from build123d import *

# Parameters (mm, degrees)
CYLINDER178_R          = 3
CYLINDER178_DEPTH      = 62
CYLINDER179_R          = 3
CYLINDER179_DEPTH      = 62
CYLINDER174_R          = 1.2
CYLINDER174_DEPTH      = 4
CYLINDER176_R          = 1.2
CYLINDER176_DEPTH      = 8
CYLINDER177_R          = 1.2
CYLINDER177_DEPTH      = 8
CYLINDER175_R          = 1.2
CYLINDER175_DEPTH      = 4
CYLINDER002_R          = 1.6
CYLINDER002_DEPTH      = 41
CYLINDER003_R          = 2.6
CYLINDER003_DEPTH      = 20
CYLINDER001_R          = 1.4
CYLINDER001_DEPTH      = 51
CYLINDER008_R          = 1.25
CYLINDER008_DEPTH      = 15
CYLINDER007_R          = 1.25
CYLINDER007_DEPTH      = 15
CYLINDER009_R          = 1.25
CYLINDER009_DEPTH      = 15
CYLINDER005_R          = 1.25
CYLINDER005_DEPTH      = 15
CYLINDER006_R          = 1.25
CYLINDER006_DEPTH      = 15
CYLINDER004_R          = 1.25
CYLINDER004_DEPTH      = 15
CYLINDER_R             = 5
CYLINDER_DEPTH         = 19
BOX084_W               = 30
BOX084_H               = 62
BOX084_DEPTH           = 10
BOX084_PLACEMENT_ANGLE = 17
BOX083_W               = 25
BOX083_H               = 42
BOX083_DEPTH           = 1.5
BOX079_W               = 25
BOX079_H               = 62
BOX079_DEPTH           = 11
FILLET045_R            = 3
BOX008_W               = 60
BOX008_H               = 60
BOX008_DEPTH           = 10
FILLET044_R            = 3
FILLET046_R            = 3


with BuildPart() as cylinder178:
    # Cylinder178 → Cylinder178 (new body)
    with BuildSketch(Plane(origin=(67, 15, 19), x_dir=(0, 0, -1), z_dir=(1, 0, 0))):
        Circle(CYLINDER178_R)
    extrude(amount=CYLINDER178_DEPTH)


with BuildPart() as fusion154:
    # Cylinder179 → Cylinder179 (new body)
    with BuildSketch(Plane(origin=(67, 47, 19), x_dir=(0, 0, -1), z_dir=(1, 0, 0))):
        Circle(CYLINDER179_R)
    extrude(amount=CYLINDER179_DEPTH)

    # Fusion154: union Cylinder178
    add(cylinder178.part)


with BuildPart() as cylinder174:
    # Cylinder174 → Cylinder174 (new body)
    with BuildSketch(Plane(origin=(50, 24, 15), x_dir=(1, 0, 0), z_dir=(0, 0, 1))):
        Circle(CYLINDER174_R)
    extrude(amount=CYLINDER174_DEPTH)


with BuildPart() as cylinder176:
    # Cylinder176 → Cylinder176 (new body)
    with BuildSketch(Plane(origin=(64, 24, 11), x_dir=(1, 0, 0), z_dir=(0, 0, 1))):
        Circle(CYLINDER176_R)
    extrude(amount=CYLINDER176_DEPTH)


with BuildPart() as cylinder177:
    # Cylinder177 → Cylinder177 (new body)
    with BuildSketch(Plane(origin=(64, 38, 11), x_dir=(1, 0, 0), z_dir=(0, 0, 1))):
        Circle(CYLINDER177_R)
    extrude(amount=CYLINDER177_DEPTH)


with BuildPart() as fusion153:
    # Cylinder175 → Cylinder175 (new body)
    with BuildSketch(Plane(origin=(50, 38, 15), x_dir=(1, 0, 0), z_dir=(0, 0, 1))):
        Circle(CYLINDER175_R)
    extrude(amount=CYLINDER175_DEPTH)

    # Fusion153: union Cylinder174, Cylinder176, Cylinder177
    add(cylinder174.part)
    add(cylinder176.part)
    add(cylinder177.part)


with BuildPart() as cylinder002:
    # Cylinder002 → Cylinder002 (new body)
    with BuildSketch(Plane(origin=(20, 31, 10), x_dir=(0, 0, -1), z_dir=(1, 0, 0))):
        Circle(CYLINDER002_R)
    extrude(amount=CYLINDER002_DEPTH)


with BuildPart() as cylinder003:
    # Cylinder003 → Cylinder003 (new body)
    with BuildSketch(Plane(origin=(41, 31, 10), x_dir=(0, 0, -1), z_dir=(1, 0, 0))):
        Circle(CYLINDER003_R)
    extrude(amount=CYLINDER003_DEPTH)


with BuildPart() as fusion149:
    # Cylinder001 → Cylinder001 (new body)
    with BuildSketch(Plane(origin=(10, 31, 10), x_dir=(0, 0, -1), z_dir=(1, 0, 0))):
        Circle(CYLINDER001_R)
    extrude(amount=CYLINDER001_DEPTH)

    # Fusion149: union Cylinder002, Cylinder003
    add(cylinder002.part)
    add(cylinder003.part)


with BuildPart() as fusion149_1:
    # Fusion149 placement: moved
    add(fusion149.part.moved(Location((-1, 0, 4))))


with BuildPart() as cylinder008:
    # Cylinder008 → Cylinder008 (new body)
    with BuildSketch(Plane(origin=(6, 15, 14), x_dir=(1, 0, 0), z_dir=(0, -1, 0))):
        Circle(CYLINDER008_R)
    extrude(amount=CYLINDER008_DEPTH)


with BuildPart() as cylinder007:
    # Cylinder007 → Cylinder007 (new body)
    with BuildSketch(Plane(origin=(28, 15, 14), x_dir=(1, 0, 0), z_dir=(0, -1, 0))):
        Circle(CYLINDER007_R)
    extrude(amount=CYLINDER007_DEPTH)


with BuildPart() as fusion008:
    # Cylinder009 → Cylinder009 (new body)
    with BuildSketch(Plane(origin=(51, 15, 14), x_dir=(1, 0, 0), z_dir=(0, -1, 0))):
        Circle(CYLINDER009_R)
    extrude(amount=CYLINDER009_DEPTH)

    # Fusion008: union Cylinder008, Cylinder007
    add(cylinder008.part)
    add(cylinder007.part)


with BuildPart() as fusion008_1:
    # Fusion008 placement: moved
    add(fusion008.part.moved(Location((0, 47, 0))))


with BuildPart() as cylinder005:
    # Cylinder005 → Cylinder005 (new body)
    with BuildSketch(Plane(origin=(6, 15, 14), x_dir=(1, 0, 0), z_dir=(0, -1, 0))):
        Circle(CYLINDER005_R)
    extrude(amount=CYLINDER005_DEPTH)


with BuildPart() as cylinder006:
    # Cylinder006 → Cylinder006 (new body)
    with BuildSketch(Plane(origin=(28, 15, 14), x_dir=(1, 0, 0), z_dir=(0, -1, 0))):
        Circle(CYLINDER006_R)
    extrude(amount=CYLINDER006_DEPTH)


with BuildPart() as fusion009:
    # Cylinder004 → Cylinder004 (new body)
    with BuildSketch(Plane(origin=(51, 15, 14), x_dir=(1, 0, 0), z_dir=(0, -1, 0))):
        Circle(CYLINDER004_R)
    extrude(amount=CYLINDER004_DEPTH)

    # Fusion007: union Cylinder005, Cylinder006
    add(cylinder005.part)
    add(cylinder006.part)

    # Fusion009: union Fusion008
    add(fusion008_1.part)


with BuildPart() as cylinder:
    # Cylinder → Cylinder (new body)
    with BuildSketch(Plane(origin=(30, 31, 6), x_dir=(1, 0, 0), z_dir=(0, 0, 1))):
        Circle(CYLINDER_R)
    extrude(amount=CYLINDER_DEPTH)


with BuildPart() as cube052:
    # Box084 → Box084 (new body)
    with BuildSketch(Plane.XY):
        with Locations((15, 31)):
            Rectangle(BOX084_W, BOX084_H)
    extrude(amount=BOX084_DEPTH)


with BuildPart() as cube052_1:
    # Box084 placement: moved
    add(cube052.part.moved(Location((-29, 0, 7))).rotate(Axis((-29, 0, 7), (0, 1, 0)), BOX084_PLACEMENT_ANGLE))


with BuildPart() as cube051:
    # Box083 → Box083 (new body)
    with BuildSketch(Plane(origin=(-24, 10, 19), x_dir=(1, 0, 0), z_dir=(0, 0, 1))):
        with Locations((12.5, 21)):
            Rectangle(BOX083_W, BOX083_H)
    extrude(amount=BOX083_DEPTH)


with BuildPart() as fillet045:
    # Box079 → Box079 (new body)
    with BuildSketch(Plane(origin=(-24, 0, 9), x_dir=(1, 0, 0), z_dir=(0, 0, 1))):
        with Locations((12.5, 31)):
            Rectangle(BOX079_W, BOX079_H)
    extrude(amount=BOX079_DEPTH)

    # Cut098: cut Cube051
    add(cube051.part, mode=Mode.SUBTRACT)

    # Fillet045
    fillet045_edges = [fillet045.edges().sort_by_distance(p)[0] for p in [
        (-11.5, 0, 20),
        (-11.5, 62, 20),
    ]]
    fillet(fillet045_edges, radius=FILLET045_R)


with BuildPart() as fifth_wheel_plate:
    # Box008 → Box008 (new body)
    with BuildSketch(Plane(origin=(0, 1, 9), x_dir=(1, 0, 0), z_dir=(0, 0, 1))):
        with Locations((30, 30)):
            Rectangle(BOX008_W, BOX008_H)
    extrude(amount=BOX008_DEPTH)

    # Fillet044
    fillet044_edges = [fifth_wheel_plate.edges().sort_by_distance(p)[0] for p in [
        (30, 1, 19),
        (30, 61, 19),
    ]]
    fillet(fillet044_edges, radius=FILLET044_R)

    # Fusion150: union Fillet045
    add(fillet045.part)

    # Cut099: cut Cube052
    add(cube052_1.part, mode=Mode.SUBTRACT)

    # Cut100: cut Cylinder
    add(cylinder.part, mode=Mode.SUBTRACT)

    # Cut101: cut Fusion009
    add(fusion009.part, mode=Mode.SUBTRACT)

    # Cut102: cut Fusion149
    add(fusion149_1.part, mode=Mode.SUBTRACT)

    # Fillet046
    fillet046_edges = [fifth_wheel_plate.edges().sort_by_distance(p)[0] for p in [
        (-1.338669, 31, 9),
        (-24, 31, 15.928264),
    ]]
    fillet(fillet046_edges, radius=FILLET046_R)


with BuildPart() as fifth_wheel_plate_1:
    # Fillet046 placement: moved
    add(fifth_wheel_plate.part.moved(Location((69, 0, 0))))

    # Cut109: cut Fusion153
    add(fusion153.part, mode=Mode.SUBTRACT)

    # Cut111: cut Fusion154
    add(fusion154.part, mode=Mode.SUBTRACT)


solid = fifth_wheel_plate_1.part
Could you check a few things on this model? Use its own coordinates, in mm. A direction names the side the tool comes from. Coordinates: 2 decimals unless noted, no trailing zeros. Loops run counter-clockwise (first coordinate to the right, second up) from the corner with the lowest first, then second, coordinate; pieces in that order, holes last.
1. Imagine slicing it at D-D (x = 112). Please give me the cut outline in (y, z).
2. Imagine slicing it at A-A (x = 85.5). Please give me the cut outline in (y, z), and give its area (3 significant figures).
3. Imagine slicing it at B-B (x = 97). Please give me the cut outline in (y, z).
4. I need wall thicknesses on L1, parallel to Y at x = 92.75, z = 14; L2, parallel to Y at x = 64, z = 14.75; L3, parallel to Y at x = 80.5, z = 14. Which ranges of each line are inside material? Lowest first, please.
5. We'd pull the mould along Z, two halves only. Please class faces 4 (the face through (98, 47, 16)), 5 (the face through (64.65, 39.01, 14.94)), 6 (the face through (109, 29, 14)), 7 (the face through (45.57, 31.43, 16.39)): released by +Z, released by -Z, zero draft, split by the parting line, or undercut.
6. For P1, Ø10, axis at x = 62.5, y = 24.5, coming from the -Z side; P2, Ø2, axis at x = 77, z = 14.5, coming from the +Y side; P3, Ø10, axis at x = 101, y = 31.5, coming from the +Z side; P4, Ø6, axis at x = 99, y = 31, coming from the +Z side, each with a flat end and sliding along its axis, tell me the tip position at first contact or that it passes through.
7. Imagine slicing it at C-C (x = 75). Please give me the cut outline in (y, z).
8. For faces 1 (the face through (76.19, 54.1, 14.38)), 2 (the face through (51.145, 38.36, 16.972)), 3 (the face through (78, 31, 14)), which set-ups out of +Z, -Z, +X, -X, +Y, -Y let a thin tool reach every point of the face, with its end or its side?
Computed values:
1. outline: (1, 9) - (61, 9) - (61, 16) arc R3 ccw to (58, 19) - (50, 19) arc R3 cw to (44, 19) - (18, 19) arc R3 cw to (12, 19) - (4, 19) arc R3 ccw to (1, 16) - close; hole circle Ø5.2 at (31, 14)
2. outline: (1, 9) - (61, 9) - (61, 16) arc R3 ccw to (58, 19) - (50, 19) arc R3 cw to (44, 19) - (18, 19) arc R3 cw to (12, 19) - (4, 19) arc R3 ccw to (1, 16) - close; hole circle Ø2.8 at (31, 14)
2. area: 562 mm2
3. outline: (1, 9) - (26.42, 9) - (26.42, 19) - (18, 19) arc R3 cw to (12, 19) - (4, 19) arc R3 ccw to (1, 16) - (1, 15.25) - (15, 15.25) - (15, 12.75) - (1, 12.75) - close; (35.58, 9) - (61, 9) - (61, 12.75) - (47, 12.75) - (47, 15.25) - (61, 15.25) - (61, 16) arc R3 ccw to (58, 19) - (50, 19) arc R3 cw to (44, 19) - (35.58, 19) - close
4. L1: y = 1 to 29.4, 32.6 to 61
4. L2: y = 0 to 22.8, 25.2 to 36.8, 39.2 to 62
4. L3: y = 1 to 29.6, 32.4 to 61
5. face 4: released by +Z
5. face 5: zero draft
5. face 6: undercut
5. face 7: released by -Z
6. P1: stops at z = 9.06
6. P2: stops at y = 61
6. P3: stops at z = 19
6. P4: passes through
7. outline: (1, 9) - (61, 9) - (61, 12.75) - (47, 12.75) - (47, 15.25) - (61, 15.25) - (61, 16) arc R3 ccw to (58, 19) - (50, 19) arc R3 cw to (44, 19) - (18, 19) arc R3 cw to (12, 19) - (4, 19) arc R3 ccw to (1, 16) - (1, 15.25) - (15, 15.25) - (15, 12.75) - (1, 12.75) - close
8. face 1: +Y
8. face 2: +Z
8. face 3: +X
